```python
from build123d import *

# Parameters (mm, degrees)
BOSS_EXTRU_1_DEPTH      = 5
ESQUISSE2_R             = 2.8575
ESQUISSE2_W             = 5
ESQUISSE2_H             = 6
ESQUISSE2_W_2           = 4.274370263
ESQUISSE2_H_2           = 8.980069935
ESQUISSE2_W_3           = 4.92
ESQUISSE2_H_3           = 3
ESQUISSE2_H_4           = 8
ESQUISSE2_H_5           = 15
ESQUISSE2_W_4           = 15
ESQUISSE2_H_6           = 5
ESQUISSE2_W_5           = 1
ESQUISSE2_H_7           = 40
ENL_V_MAT_EXTRU_1_DEPTH = 5
ESQUISSE3_W             = 5
ESQUISSE3_H             = 5
BOSS_EXTRU_2_DEPTH      = 5


with BuildPart() as part:
    # Esquisse1 → Boss.-Extru.1 (new body)
    with BuildSketch(Plane.XY):
        Polygon((65.121094869, 0), (30.122364869, 0), (30.122364869, 3), (35.122364869, 3), (35.122364869, 8), (30.122364869, 8), (30.122364869, 10), (55.617614869, 10), (55.617614869, 50.2), (30.122364869, 50.2), (30.122364869, 52.2), (35.122364869, 52.2), (35.122364869, 57.2), (30.122364869, 57.2), (30.122364869, 62.2), (33.512280837, 62.2), (33.512280837, 78.240708175), (55.911629737, 78.240708175), (55.911629737, 101.750434868), (52.693, 101.750434868), (52.693, 122.246954868), (12.493, 122.246954868), (12.493, 101.750434868), (-2.878905131, 101.750434868), (-2.878905131, 153), (24.121094869, 180), (24.121094869, 260), (0, 260), (0, 270), (65.121094869, 270), align=None)
    extrude(amount=-BOSS_EXTRU_1_DEPTH)

    # Esquisse2 → Enlèv. mat.-Extru.1 (cut)
    with BuildSketch(Plane.XY):
        with Locations((12.493, 119.389454868)):
            Circle(ESQUISSE2_R)
        with Locations((32.622364869, 144.401636706)):
            Rectangle(ESQUISSE2_W, ESQUISSE2_H)
        with Locations((32.622364869, 130.246954868)):
            Rectangle(ESQUISSE2_W, ESQUISSE2_H)
        with Locations((58.048814869, 97.260399901)):
            Rectangle(ESQUISSE2_W_2, ESQUISSE2_H_2)
        with Locations((62.661094869, 1.5)):
            Rectangle(ESQUISSE2_W_3, ESQUISSE2_H_3)
        with Locations((62.661094869, 62)):
            Rectangle(ESQUISSE2_W_3, ESQUISSE2_H_4)
        with Locations((62.661094869, 168.5)):
            Rectangle(ESQUISSE2_W_3, ESQUISSE2_H_5)
        with Locations((62.661094869, 138.5)):
            Rectangle(ESQUISSE2_W_3, ESQUISSE2_H_5)
        with Locations((62.661094869, 198.5)):
            Rectangle(ESQUISSE2_W_3, ESQUISSE2_H_5)
        with Locations((62.661094869, 228.5)):
            Rectangle(ESQUISSE2_W_3, ESQUISSE2_H_5)
        with Locations((62.661094869, 258.5)):
            Rectangle(ESQUISSE2_W_3, ESQUISSE2_H_5)
        with Locations((47.621094869, 267.5)):
            Rectangle(ESQUISSE2_W_4, ESQUISSE2_H_6)
        with Locations((17.621094869, 267.5)):
            Rectangle(ESQUISSE2_W_4, ESQUISSE2_H_6)
        with Locations((24.621094869, 240)):
            Rectangle(ESQUISSE2_W_5, ESQUISSE2_H_7)
    extrude(amount=-ENL_V_MAT_EXTRU_1_DEPTH, mode=Mode.SUBTRACT)

    # Esquisse3 → Boss.-Extru.2 (add)
    with BuildSketch(Plane.XY):
        with Locations((1.993, 99.250434868)):
            Rectangle(ESQUISSE3_W, ESQUISSE3_H)
    extrude(amount=-BOSS_EXTRU_2_DEPTH)


solid = part.part
```
Input: part model. Units: mm. Frame: model coordinates. A direction names the side the tool comes from. Round coordinates to 2 decimals unless told otherwise and drop trailing zeros. Loops run counter-clockwise (first coordinate to the right, second up) from the corner with the lowest first, then second, coordinate; pieces in that order, holes last. Notation, with made-up numbers: (0, 51.5) -> (17, 51.5) arc R24 ccw to (17, 85.5) -> close; hole circle Ø9 at (67.5, 58.5). An arc over 180 degrees is marked (long way). Write each question's results on one line, items separated by ' | '.
1. Mould query, pull axis Y, two halves, no side actions, for faces 4 (the face through (63, 58, -2)), 5 (the face through (25.121, 267, -2)), 6 (the face through (45, 0, -2)), 7 (the face through (33, 122.247, -2)). Classes: +Y half, -Y half, draft (parallel to the pull), parting line (faces both ways), or undercut.
Geometry results:
face 4: undercut | face 5: draft | face 6: -Y half | face 7: undercut
2. Section A-A (x = 37.5). Return loops of the section in (y, z).
Geometry results:
outline: (0, -5) -> (10, -5) -> (10, 0) -> (0, 0) -> close; (50.2, -5) -> (78.24, -5) -> (78.24, 0) -> (50.2, 0) -> close; (122.25, -5) -> (270, -5) -> (270, 0) -> (122.25, 0) -> close
3. Section B-B (y = 47.5). Return loops of the section in (x, z).
Geometry results:
outline: (55.62, -5) -> (65.12, -5) -> (65.12, 0) -> (55.62, 0) -> close
4. Section C-C (z = -2.6). State how many separate pieces and enclosed holes the cut face has, and give its area (3 significant figures).
Geometry results:
separate pieces: 1 | enclosed holes: 2 | area: 9,190 mm2
5. Section D-D (y = 248). Return loops of the section in (x, z).
Geometry results:
outline: (25.12, -5) -> (65.12, -5) -> (65.12, 0) -> (25.12, 0) -> close
6. Ray query, line 1 (Y direction, x = 46, z = -1.85); line 2 (Y direction, x = 36.5, z = -4.5); line 3 (Y direction, x = 25, z = -3.85). Return the intervals inside material, ascending. Write a range as from..to.
Geometry results:
line 1: 0..10, 50.2..78.24, 122.25..265 | line 2: 0..10, 50.2..78.24, 122.25..270 | line 3: 122.25..220, 260..265
7. Set-up query: faces 1 (the face through (63, 266, -2)), 2 (the face through (30.122, 144, -2)), 3 (the face through (33, 52.2, -2)). Return all of +Z, -Z, +X, -X, +Y, -Y with unobstructed straight access to the full face (end or side cutting, diameter ignored); none if empty.
Geometry results:
face 1: +Z, -Z, +X | face 2: +Z, -Z | face 3: +Z, -Z, -X
8. First-contact query: P1, Ø0.7, axis at x = -1.5, z = -1.5, coming from the -Y side; P2, Ø2.5, axis at y = 87, z = -1.5, coming from the -X side; P3, Ø2.5, axis at y = 5, z = -2.5, coming from the -X side. Flat tips, straight axial feed; report the tip coordinate or a pass-through.
Geometry results:
P1: y = 101.75 | P2: x = 55.91 | P3: x = 35.12
